Check sheet for the modelled part. Datum: model origin and axes. Units: mm. A direction names the side the tool comes from. Give positions to 0.01 mm unless a question says otherwise; leave off trailing zeros. Order: outer loops, then holes, each group sorted by start corner. A loop starts at its lowest first (then second) coordinate and runs counter-clockwise, first axis right, second up. Notation, with made-up numbers: M 22.25,-16 L 69.25,-16 A21 ccw 69.25,-6 Z; hole C 86,-24 d11. An arc over 180 degrees is marked long. One line per question, with ' | ' between items. Start each with the question number.
```python
from build123d import *

# Parameters (mm, degrees)
SKETCH1_W           = 87.47
SKETCH1_H           = 70
BOSS_EXTRUDE1_DEPTH = 7.6
SKETCH2_R           = 43.735
BOSS_EXTRUDE2_DEPTH = 12
SKETCH3_R           = 51.735
BOSS_EXTRUDE3_DEPTH = 12
SKETCH4_R           = 35
CUT_EXTRUDE1_DEPTH  = 12
FILLET1_R           = 3.8
FILLET2_R           = 3.8


with BuildPart() as part:
    # Sketch1 → Boss-Extrude1 (new body)
    with BuildSketch(Plane(origin=(0, 0, 0), x_dir=(1, 0, 0), z_dir=(0, 1, 0))):
        with Locations((43.735, 35)):
            Rectangle(SKETCH1_W, SKETCH1_H)
    extrude(amount=BOSS_EXTRUDE1_DEPTH)

    # Sketch2 → Boss-Extrude2 (add)
    with BuildSketch(Plane(origin=(0, 7.6, 0), x_dir=(1, 0, 0), z_dir=(0, 1, 0))):
        with Locations(Location((43.735, 0, 0), (0, 0, 270))):
            Circle(SKETCH2_R)
    extrude(amount=-BOSS_EXTRUDE2_DEPTH)

    # Sketch3 → Boss-Extrude3 (add)
    with BuildSketch(Plane(origin=(0, 7.6, 0), x_dir=(1, 0, 0), z_dir=(0, 1, 0))):
        with Locations(Location((43.735, 0, 0), (0, 0, 270))):
            Circle(SKETCH3_R)
    extrude(amount=-BOSS_EXTRUDE3_DEPTH)

    # Sketch4 → Cut-Extrude1 (cut)
    with BuildSketch(Plane(origin=(0, 7.6, 0), x_dir=(1, 0, 0), z_dir=(0, 1, 0))):
        with Locations(Location((43.735, 0, 0), (0, 0, 270))):
            Circle(SKETCH4_R)
    extrude(amount=-CUT_EXTRUDE1_DEPTH, mode=Mode.SUBTRACT)

    # Fillet1
    fillet1_edges = [part.edges().sort_by_distance(p)[0] for p in [
        (87.47, 0, -48.818104067),
        (87.47, 7.6, -48.818104067),
        (0, 7.6, -48.818104067),
        (0, 0, -48.818104067),
    ]]
    fillet(fillet1_edges, radius=FILLET1_R - 0.0001)  # a hair under: the kernel refuses the full size

    # Fillet2
    fillet2_edges = [part.edges().sort_by_distance(p)[0] for p in [
        (43.735, 7.6, -70),
        (43.735, 0, -70),
        (86.357035058, 6.487035058, -70),
        (86.357035058, 1.112964942, -70),
        (1.112964942, 1.112964942, -70),
        (1.112964942, 6.487035058, -70),
    ]]
    fillet(fillet2_edges, radius=FILLET2_R - 0.0001)  # a hair under: the kernel refuses the full size


solid = part.part
```
Item 1: Section check A-A, the plane z = 0. Record the cut outline in (x, y) (3 decimals).
Item 2: Set-up check for faces 1 (the face through (86.327, 6.516, -47.188)), 2 (the face through (86.386, 1.143, -47.188)), 3 (the face through (1.143, 1.084, -47.188)): record each of +Z, -Z, +X, -X, +Y, -Y from which the full face is reachable in a straight line by a thin tool's end or side.
Item 3: Section check C-C, the plane y = 6.25. Record the cut outline in (x, z) (3 decimals), then the cut area to 3 significant figures.
Item 4: Draft check along Z on faces 4 (the face through (22.438, 1.684, -27.775)), 5 (the face through (59.275, 1.684, 49.346)), 6 (the face through (43.176, 1.143, -68.916)), 7 (the face through (33, -4.4, 34)). Enter one of: released by +Z, released by -Z, zero draft, split by the parting line, or undercut.
Item 5: Go/stop test with flat-tipped pins: P1, Ø4, axis at y = 1, z = 0, coming from the -X side; P2, Ø2, axis at x = 66.5, y = 1, coming from the +Z side; P3, Ø2, axis at x = 2.5, y = 2, coming from the -Z side; P4, Ø8, axis at x = 58.5, z = -50.5, coming from the -Y side. Record where each tip stops, or that it passes through.
Item 6: Section check D-D, the plane z = 21. Record the cut outline in (x, y) (3 decimals), then the cut area to 3 significant figures.
Item 7: Scan lines: probe 1 along X at (y, z) = (1.25, 0) (3 decimals); probe 2 along X at (y, z) = (2, -17.5); probe 3 along Z at (x, y) = (65.5, 4.5). Record each from-to range of solid material in increasing order. Write a range as [from, to].
Reported:
1) outline: M -8,-4.4 L 8.735,-4.4 L 8.735,7.6 L -8,7.6 Z; M 78.735,-4.4 L 95.47,-4.4 L 95.47,7.6 L 78.735,7.6 Z
2) face 1: -Z, +X, +Y | face 2: -Z, +X, -Y | face 3: -Z, -X, -Y
3) outline: M 0.895,-66.2 A2.905 ccw 3.8,-69.105 L 83.67,-69.105 A2.905 ccw 86.575,-66.2 L 86.575,-29.005 A51.735 ccw long 0.895,-29.005 Z; hole C 43.735,0 d70 | area: 6,620 mm^2
4) face 4: undercut | face 5: split by the parting line | face 6: released by -Z | face 7: zero draft
5) P1: stops at x = -8 | P2: stops at z = 46.93 | P3: stops at z = -69.8 | P4: stops at y = -4.4
6) outline: M -3.546,-4.4 L 15.735,-4.4 L 15.735,7.6 L -3.546,7.6 Z; M 71.735,-4.4 L 91.016,-4.4 L 91.016,7.6 L 71.735,7.6 Z | area: 463 mm^2
7) probe 1: x = [-8, 8.735], [78.735, 95.47] | probe 2: x = [-4.95, 13.42], [74.05, 92.42] | probe 3: z = [-69.93, -27.41], [27.41, 46.93]
